For this review, take the finished solid that the model builds, in its own axes (mm). A direction names the side the tool comes from. Coordinates: 2 decimals unless noted, no trailing zeros. Loops run counter-clockwise (first coordinate to the right, second up) from the corner with the lowest first, then second, coordinate; pieces in that order, holes last. Notation, with made-up numbers: M 32,74 L 87,74 A24 cw 87,102 Z; hole C -25,41.25 d5. An arc over 180 degrees is marked long. Answer as a JSON object with one key per item and string values. Group by question number.
Item 1: Wall thickness on L1, parallel to Z at x = -60, y = 77.25; L2, parallel to Y at x = 8, z = 9.5; L3, parallel to Y at x = -6, z = 26: over which ranges is each line inside the solid? List them lowest first. Write a range as from..to.
Item 2: Mouldability with a two-part tool opening along X and no side actions: class faces 1 (the face through (-1, 1, 2.5)), 2 (the face through (2.2, -74.9, 50)), 3 (the face through (95.38, 30.04, 24.65)) as +X half, -X half, draft (parallel to the pull), parting line (faces both ways), or undercut.
Item 3: Add section B-B (x = -60). State the section outline as (y, z) points, then the cut area to 3 significant figures.
Item 4: Add section A-A (z = 25). Count the separate pieces of the cut face and the enclosed holes in it, then the cut area to 3 significant figures.
Item 5: Add section D-D (y = -25). State the section outline as (x, z) points, then the cut area to 3 significant figures.
Item 6: Insertion check: pin 1 (6 mm diameter, centred on y = -25.5, z = 5, fed in from -X); pin 2 (2 mm diameter, centred on x = -56.5, z = 28.5, fed in from +Y); pin 3 (1.5 mm diameter, centred on y = 2.5, z = 39, fed in from -X). Each pin has a flat end and moves straight along its axis. Give the tip position at first contact, or say it passes through.
Item 7: Add section C-C (x = -17.5). State the section outline as (y, z) points, then the cut area to 3 significant figures.
Item 8: Tool access review of faces 4 (the face through (74.9, -2.2, 50)), 5 (the face through (-25, 60, 27)), 6 (the face through (-60.796, 78.069, 44.936)): name each direction out of +Z, -Z, +X, -X, +Y, -Y from which nothing blocks a thin tool from reaching the whole face with its end or side.
from build123d import *

# Parameters (mm, degrees)
F0_R     = 100
F1_DEPTH = 50
F2_T     = -2.5
F3_R     = 5
F3_R_2   = 2
F4_DEPTH = 47.5
F6_R     = 5
F7_DEPTH = 100.001
F5_W     = 50
F5_H     = 10
F8_DEPTH = 47.5


with BuildPart() as f1:
    # F0 (on Top) → F1 (new body)
    with BuildSketch(Plane.XY):
        Circle(F0_R)
    extrude(amount=F1_DEPTH)

    # F2
    f2_openings = [f1.faces().sort_by_distance(p)[0] for p in [
        (0, 0, 50),
    ]]
    offset(amount=F2_T, openings=f2_openings)

    # F3 (on face) → F4 (join, through all)
    with BuildSketch(Plane.XY.offset(50)):
        with Locations((-75, 0)):
            Circle(F3_R)
        with Locations((-75, 0)):
            Circle(F3_R_2, mode=Mode.SUBTRACT)
        with Locations((0, -75)):
            Circle(F3_R)
        with Locations((0, -75)):
            Circle(F3_R_2, mode=Mode.SUBTRACT)
        with Locations((75, 0)):
            Circle(F3_R)
        with Locations((75, 0)):
            Circle(F3_R_2, mode=Mode.SUBTRACT)
        with Locations((0, 75)):
            Circle(F3_R)
        with Locations((0, 75)):
            Circle(F3_R_2, mode=Mode.SUBTRACT)
    extrude(amount=-F4_DEPTH)

    # F6 (on Front) → F7 (cut, through all)
    with BuildSketch(Plane.XZ):
        with Locations((-60, 40)):
            Circle(F6_R)
    extrude(amount=-F7_DEPTH, mode=Mode.SUBTRACT)

    # F5 (on face) → F8 (join, through all)
    with BuildSketch(Plane.XY.offset(50)):
        with Locations((0, 60)):
            Rectangle(F5_W, F5_H)
    extrude(amount=-F8_DEPTH)


solid = f1.part
From the geometry:
{
 "1": {"L1": "z = 0..35, 45..50", "L2": "y = -99.68..-97.17, 55..65, 97.17..99.68", "L3": "y = -99.82..-97.32, 55..65, 97.32..99.82"},
 "2": {"face 1": "undercut", "face 2": "draft", "face 3": "parting line"},
 "3": {"outline": "M -80,0 L 80,0 L 80,35 L 76.85,35 L 76.85,2.5 L -76.85,2.5 L -76.85,50 L -80,50 Z; M 76.85,45 L 80,45 L 80,50 L 76.85,50 Z", "area": "668 mm²"},
 "4": {"separate pieces": "6", "enclosed holes": "5", "area": "2,320 mm²"},
 "5": {"outline": "M -96.82,0 L 96.82,0 L 96.82,50 L 94.24,50 L 94.24,2.5 L -94.24,2.5 L -94.24,50 L -96.82,50 Z", "area": "730 mm²"},
 "6": {"pin 1": "stops at x = -97.44", "pin 2": "stops at y = 83.19", "pin 3": "stops at x = -99.98"},
 "7": {"outline": "M -98.46,0 L 98.46,0 L 98.46,50 L 95.92,50 L 95.92,2.5 L 65,2.5 L 65,50 L 55,50 L 55,2.5 L -95.92,2.5 L -95.92,50 L -98.46,50 Z", "area": "1,210 mm²"},
 "8": {"face 4": "+Z, +X, -X, +Y, -Y", "face 5": "+Z", "face 6": "+Y"}
}
